```python
from build123d import *

# Parameters (mm, degrees)
F0_W     = 5
F0_H     = 5
F0_W_2   = 12.8715214133
F0_H_2   = 2.8254000843
F1_DEPTH = 25
F2_R     = 4.99999


# Not quite as in the source:
# - a fillet or chamfer is up to 0.001 mm smaller than in the source, because OpenCascade refuses the exact size


with BuildPart() as f1:
    # F0 (on Top) → F1 (new body)
    with BuildSketch(Plane.XY):
        with Locations((2.5, -2.5)):
            Rectangle(F0_W, F0_H)
        with Locations((11.4357607067, -2.5)):
            Rectangle(F0_W_2, F0_H)
        Polygon((5, -5), (0, -5), (0, -25), (5, -25), (5, -22.1745999157), align=None)
        with Locations((7.5, -23.5872999579)):
            Rectangle(F0_W, F0_H_2)
        Polygon((10, -10), (10, -22.1745999157), (10, -25), (15, -25), (15, -10), align=None)
    extrude(amount=F1_DEPTH)

    # F2 (radius 5 in the source; OpenCascade refuses exactly that, so slightly less here)
    f2_edges = [f1.edges().sort_by_distance(p)[0] for p in [
        (0, 0, 12.5),
        (0, -25, 12.5),
        (15, -25, 12.5),
        (17.871521, 0, 12.5),
    ]]
    fillet(f2_edges, radius=F2_R)


solid = f1.part
```
CAD build for the part. Positions are in the model's coordinates, mm. A direction names the side the tool comes from. Round coordinates to 2 decimals unless told otherwise and drop trailing zeros. Write each loop counter-clockwise with the first axis right and the second up, starting at its lowest first coordinate (ties: lowest second). Pieces come first, ordered by that corner, then holes. Notation, with made-up numbers: (56.25, -39) -> (67.25, -39) arc R13 cw to (67.25, -17) -> close; hole circle Ø11 at (-33.5, 83.25). An arc over 180 degrees is marked (long way). Answer in a Markdown table with one row per item. Add a question column.
Item 1: Drop flat-ended pins along their axis: pin 1 Ø11 at (y, z) = (-14, 10.5) entering from +X; pin 2 Ø1 at (x, y) = (13.5, -7) entering from -Z. Give the stop position or say it passes through.
Item 2: Mould opens along X. For faces 1 (the face through (11, -5, 12)), 2 (the face through (16.446, -1.504, 12.675)), 3 (the face through (7, -22.175, 12)), 4 (the face through (1, -23, 13)) say: pulls with the +X half, pulls with the -X half, needs draft (parallel to the pull), parting line crosses it, or undercut.
Item 3: Saw through at A-A, the plane x = 8.25. Write the cut outline in (y, z).
Item 4: Saw through at B-B, the plane y = -13.25. Write the cut outline in (x, z).
Item 5: Drill centre lines: line 1 (X direction, y = -11, z = 15.5); line 2 (Y direction, x = 5.5, z = 13); line 3 (X direction, y = -8.5, z = 20.75). Where is each one in solid material? Low to high. Write a range as from..to.
Item 6: Which spindle directions (+Z, -Z, +X, -X, +Y, -Y) get a long thin tool onto all of the face, cutting with end or side? Do faces 5 (the face through (13, -10, 12)), 6 (the face through (5, -14, 12)), 7 (the face through (15, -15, 12)). Say none if no direction does.
Item 7: Saw through at D-D, the plane y = -5.75. Write the cut outline in (x, z), then the cut area to 3 significant figures.
Findings below:
| question | item | result |
|---|---|---|
| 1 | pin 1 | stops at x = 15 |
| 1 | pin 2 | passes through |
| 2 | face 1 | needs draft |
| 2 | face 2 | pulls with the +X half |
| 2 | face 3 | undercut |
| 2 | face 4 | pulls with the -X half |
| 3 | outline | (-25, 0) -> (-22.17, 0) -> (-22.17, 25) -> (-25, 25) -> close; (-5, 0) -> (0, 0) -> (0, 25) -> (-5, 25) -> close |
| 4 | outline | (0, 0) -> (5, 0) -> (5, 25) -> (0, 25) -> close; (10, 0) -> (15, 0) -> (15, 25) -> (10, 25) -> close |
| 5 | line 1 | x = 0..5, 10..15 |
| 5 | line 2 | y = -25..-22.17, -5..0 |
| 5 | line 3 | x = 0..5 |
| 6 | face 5 | +Z, -Z, +X |
| 6 | face 6 | +Z, -Z |
| 6 | face 7 | +Z, -Z, +X, -Y |
| 7 | outline | (0, 0) -> (5, 0) -> (5, 25) -> (0, 25) -> close |
| 7 | area | 125 mm^2 |
